```python
from build123d import *

# Parameters (mm, degrees)
SKETCH1_R           = 4.7625
SKETCH1_R_2         = 1.5875
BOSS_EXTRUDE1_DEPTH = 3.96875
CHAMFER1_SIZE       = 0.2
FILLET1_R           = 0.25


with BuildPart() as part:
    # Sketch1 → Boss-Extrude1 (new body)
    with BuildSketch(Plane(origin=(0, 0, 0), x_dir=(0, 0, -1), z_dir=(1, 0, 0))):
        Circle(SKETCH1_R)
        Circle(SKETCH1_R_2, mode=Mode.SUBTRACT)
    extrude(amount=BOSS_EXTRUDE1_DEPTH)

    # Chamfer1
    chamfer1_edges = [part.edges().sort_by_distance(p)[0] for p in [
        (0, 0, 1.5875),
        (3.96875, 0, 1.5875),
    ]]
    chamfer(chamfer1_edges, length=CHAMFER1_SIZE)

    # Fillet1
    fillet1_edges = [part.edges().sort_by_distance(p)[0] for p in [
        (0, 0, 4.7625),
        (3.96875, 0, 4.7625),
    ]]
    fillet(fillet1_edges, radius=FILLET1_R)


solid = part.part
```
The model under review builds one solid part; all positions refer to its coordinate system, in mm. Round coordinates to 2 decimals unless told otherwise and drop trailing zeros. Write each loop counter-clockwise with the first axis right and the second up, starting at its lowest first coordinate (ties: lowest second). Pieces come first, ordered by that corner, then holes. Notation, with made-up numbers: (41.5, 41.5) -> (88.5, 41.5) arc R20 cw to (88.5, 55.5) -> close; hole circle Ø6 at (27, 28). An arc over 180 degrees is marked (long way). Use CSV: the item, a comma, the result in double quotes.
Q1. For pin 1 Ø2 at (x, z) = (1, 1.5) entering from -Y, flat-tipped, find the tip position at first contact; note if it passes through.
Checks:
pin 1,"y = -4.74"
Q2. Consider section A-A (y = 0). Give the boundary of the cut face in (x, z), then the cut area to 3 significant figures.
Checks:
outline,"(0, -4.51) arc R0.25 ccw to (0.25, -4.76) -> (3.72, -4.76) arc R0.25 ccw to (3.97, -4.51) -> (3.97, -1.79) -> (3.77, -1.59) -> (0.2, -1.59) -> (0, -1.79) -> close; (0, 1.79) -> (0.2, 1.59) -> (3.77, 1.59) -> (3.97, 1.79) -> (3.97, 4.51) arc R0.25 ccw to (3.72, 4.76) -> (0.25, 4.76) arc R0.25 ccw to (0, 4.51) -> close"
area,"25.1 mm²"
Q3. Consider section C-C (x = 1.1). Give the boundary of the cut face in (y, z) (1 decimal), then the cut area to 3 significant figures.
Checks:
outline,"circle Ø9.5 at (0, 0); hole circle Ø3.2 at (0, 0)"
area,"63.3 mm²"
Q4. To check wall thickness, follow probe 1 along Y at (x, z) = (1.15, 0); probe 2 along Y at (x, z) = (2, 0.5); probe 3 along Z at (x, y) = (1.9, -3.75). State the ranges of each line that lie inside material, in increasing order. Write a range as [from, to].
Checks:
probe 1,"[-4.76, -1.59], [1.59, 4.76]"
probe 2,"[-4.74, -1.51], [1.51, 4.74]"
probe 3,"[-2.94, 2.94]"
Q5. Mouldability with a two-part tool opening along Y and no side actions: class faces 1 (the cylindrical face through (1.96, -2.9, 3.78)), 2 (the flat face through (3.969, -2, 0)), 3 (the cylindrical face through (1.96, -1.55, 0.34)) as released by +Y, released by -Y, zero draft, split by the parting line, or undercut.
Checks:
face 1,"split by the parting line"
face 2,"zero draft"
face 3,"undercut"
